Can you work these out from the drawing? Everything is in mm from the part's minimum corner. A direction names the side the tool comes from. Give positions to 0.01 mm unless a question says otherwise; leave off trailing zeros. Write each loop counter-clockwise with the first axis right and the second up, starting at its lowest first coordinate (ties: lowest second). Pieces come first, ordered by that corner, then holes. Notation, with made-up numbers: (73, 49) -> (110, 49) arc R19 ccw to (110, 86) -> close; hole circle Ø1 at (25, 75.25). An arc over 180 degrees is marked (long way). Answer as CSV lines item,"result". Start each with the question number.
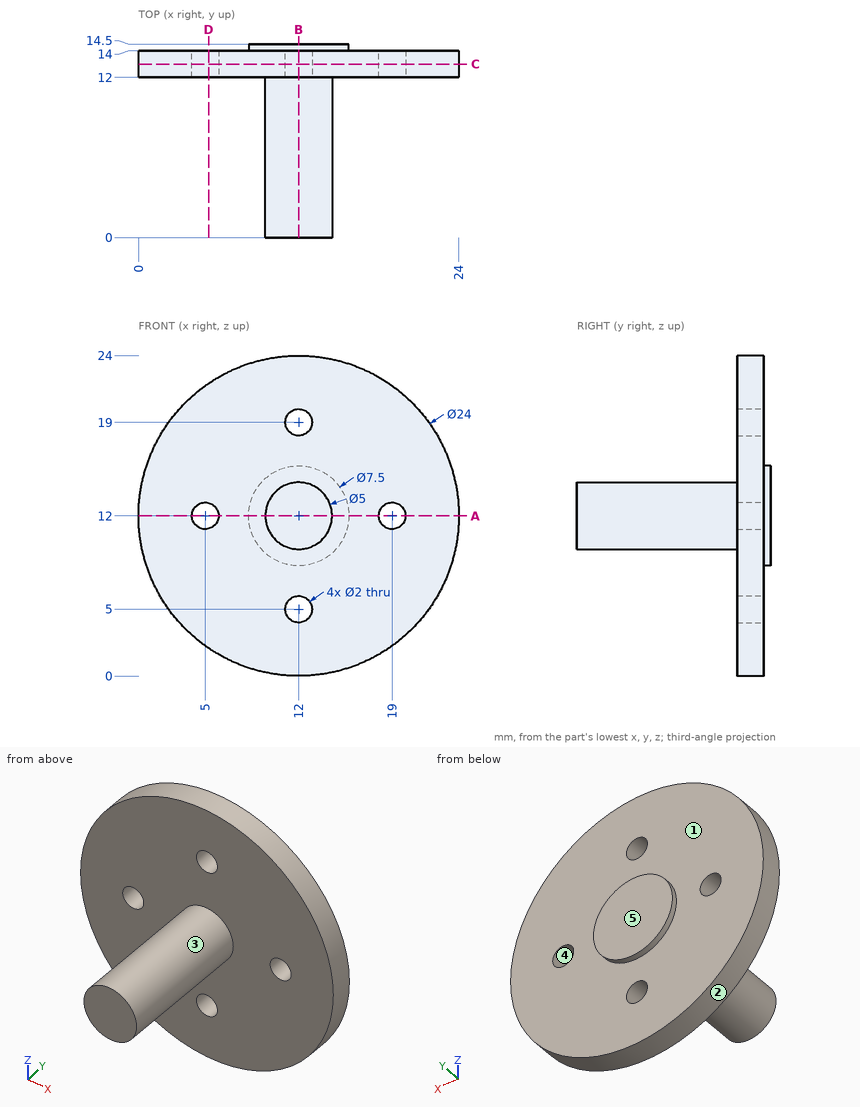
Item 1: For the marked faces 1 and 2, which set-ups out of +Z, -Z, +X, -X, +Y, -Y let a thin tool reach every point of the face, with its end or its side?
Item 2: If I drill on line 1 (Z direction, x = 12, y = 12.65); line 2 (Y direction, x = 21, z = 15.75); line 3 (Z direction, x = 5, y = 13.2), over which ranges is the centre line in solid material (lowest first)? Write a range as [from, to].
Item 3: If we section it at A-A (z = 12): Please give me the cut outline in (x, y).
Item 4: I'm going to push flat-ended pins straight in: pin 1 (1.8 mm diameter, centred on x = 19, z = 12, fed in from +Y); pin 2 (4 mm diameter, centred on x = 11.5, y = 2.5, fed in from -Z); pin 3 (3 mm diameter, centred on x = 16, y = 11, fed in from +Z); pin 4 (2 mm diameter, centred on x = 18, z = 13.5, fed in from +Y). Where does each tip first touch, or does it pass through?
Item 5: We'd pull the mould along X, two halves only. Please class the marked faces 3, 4 and 5: released by +X, released by -X, zero draft, split by the parting line, or undercut.
Item 6: If we section it at C-C (y = 13): Please give me the cut outline in (x, z), and give its area (3 significant figures).
Item 7: If we section it at B-B (x = 12): Please give me the cut outline in (y, z).
Item 8: If we section it at D-D (x = 5.25): Please give me the cut outline in (y, z).
Final values:
1,face 1,"+Y"
1,face 2,"+Y, -Y"
2,line 1,"[0, 4], [6, 18], [20, 24]"
2,line 2,"[12, 14]"
2,line 3,"[2.25, 11], [13, 21.75]"
3,outline,"(0, 12) -> (4, 12) -> (4, 14) -> (0, 14) -> close; (6, 12) -> (9.5, 12) -> (9.5, 0) -> (14.5, 0) -> (14.5, 12) -> (18, 12) -> (18, 14) -> (15.75, 14) -> (15.75, 14.5) -> (8.25, 14.5) -> (8.25, 14) -> (6, 14) -> close; (20, 12) -> (24, 12) -> (24, 14) -> (20, 14) -> close"
4,pin 1,"through"
4,pin 2,"z = 9.5"
4,pin 3,"z = 23.65"
4,pin 4,"y = 14"
5,face 3,"split by the parting line"
5,face 4,"undercut"
5,face 5,"zero draft"
6,outline,"circle Ø24 at (12, 12); hole circle Ø2 at (5, 12); hole circle Ø2 at (12, 5); hole circle Ø2 at (12, 19); hole circle Ø2 at (19, 12)"
6,area,"440 mm2"
7,outline,"(0, 9.5) -> (12, 9.5) -> (12, 6) -> (14, 6) -> (14, 8.25) -> (14.5, 8.25) -> (14.5, 15.75) -> (14, 15.75) -> (14, 18) -> (12, 18) -> (12, 14.5) -> (0, 14.5) -> close; (12, 0) -> (14, 0) -> (14, 4) -> (12, 4) -> close; (12, 20) -> (14, 20) -> (14, 24) -> (12, 24) -> close"
8,outline,"(12, 2.08) -> (14, 2.08) -> (14, 11.03) -> (12, 11.03) -> close; (12, 12.97) -> (14, 12.97) -> (14, 21.92) -> (12, 21.92) -> close"
